Check sheet for the modelled part. Datum: model origin and axes. Units: mm. Face numbers are marked on the shaded views. Coordinates: 2 decimals unless noted, no trailing zeros. Loops run counter-clockwise (first coordinate to the right, second up) from the corner with the lowest first, then second, coordinate; pieces in that order, holes last. Notation, with made-up numbers: M 38,33.25 L 80,33.25 A19 cw 80,48.25 Z; hole C 65,49.25 d10. An arc over 180 degrees is marked long. Use CSV: the item, a comma, the result in double quotes. Start each with the question number.
(1) Go/stop test with flat-tipped pins: pin 1 Ø10 at (x, z) = (31.5, 4.5) entering from -Y; pin 2 Ø1 at (x, z) = (12.5, 5.5) entering from -Y; pin 3 Ø5 at (y, z) = (-11, 4) entering from +X. Record where each tip stops, or that it passes through.
(2) Scan lines: line 1 (Y direction, x = 17.5, z = -7.35); line 2 (Y direction, x = 17.5, z = -1.25); line 3 (X direction, y = -21, z = 1.5). Record each from-to range of solid material in increasing order.
(3) Draft check along Y on the marked faces 1, 2 and 3. Enter one of: pulls with the +Y half, pulls with the -Y half, needs draft (parallel to the pull), parting line crosses it, or undercut.
(4) Section check A-A on z = -7.5. Record the cut outline in (x, y), and give its area (3 significant figures).
from build123d import *

# Parameters (mm, degrees)
F0_W      = 35
F0_H      = 35
F2_W      = 25
F2_H      = 25
F4_W      = 35
F4_H      = 35
F4_R      = 1.6
F5_DEPTH  = 10
F6_DEPTH  = 10.0010001
F7_R      = 4
F7_R_2    = 1.6
F8_DEPTH  = 15
F10_DEPTH = 25


with BuildPart() as f3:
    # F0 (on Top) → F3 section 0
    with BuildSketch(Plane.XY):
        with Locations((17.5, -17.5)):
            Rectangle(F0_W, F0_H)
    # F2 (on offset) → F3 section 1
    with BuildSketch(Plane.XY.offset(10)):
        with Locations((12.5, -12.5)):
            Rectangle(F2_W, F2_H)
    loft()

    # F4 (on face) → F5 (join)
    with BuildSketch(Plane(origin=(0, 0, 0), x_dir=(1, 0, 0), z_dir=(0, 0, -1))):
        with Locations((17.5, 17.5)):
            Rectangle(F4_W, F4_H)
        with Locations((17.5, 17.5)):
            Circle(F4_R, mode=Mode.SUBTRACT)
    extrude(amount=F5_DEPTH)

    # F4 (on face) → F6 (cut, through all)
    with BuildSketch(Plane(origin=(0, 0, 0), x_dir=(1, 0, 0), z_dir=(0, 0, -1))):
        with Locations((17.5, 17.5)):
            Circle(F4_R)
    extrude(amount=-F6_DEPTH, mode=Mode.SUBTRACT)

    # F7 (on face) → F8 (cut)
    with BuildSketch(Plane.XY.offset(10)):
        with Locations((17.5, -17.5)):
            Circle(F7_R)
        with Locations((17.5, -17.5)):
            Circle(F7_R_2, mode=Mode.SUBTRACT)
    extrude(amount=-F8_DEPTH, mode=Mode.SUBTRACT)

    # F9 (on face) → F10 (cut)
    with BuildSketch(Plane(origin=(0, 0, -10), x_dir=(1, 0, 0), z_dir=(0, 0, -1))):
        Polygon((35, 25), (35, 35), (25, 35), align=None)
    extrude(amount=-F10_DEPTH, mode=Mode.SUBTRACT)


solid = f3.part
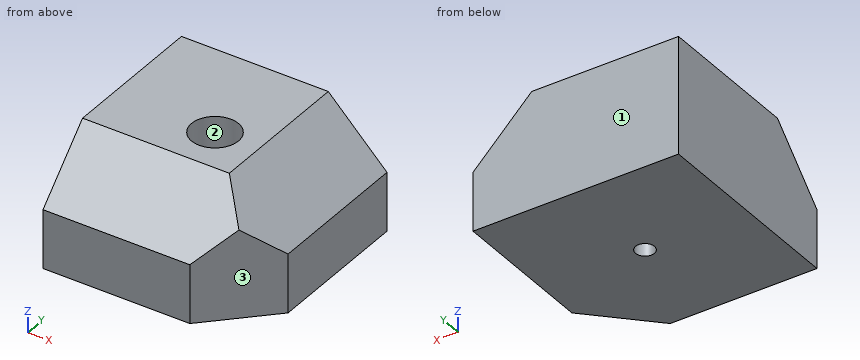
Outcome:
1,pin 1,"stops at y = -32.89"
1,pin 2,"stops at y = -30"
1,pin 3,"stops at x = 33.5"
2,line 1,"y = -35 to -19.1, -15.9 to 0"
2,line 2,"y = -35 to -21.5, -13.5 to 0"
2,line 3,"x = 0 to 15.56, 19.44 to 33.5"
3,face 1,"pulls with the +Y half"
3,face 2,"undercut"
3,face 3,"pulls with the -Y half"
4,outline,"M 0,-35 L 25,-35 L 35,-25 L 35,0 L 0,0 Z; hole C 17.5,-17.5 d3.2"
4,area,"1,170 mm²"
